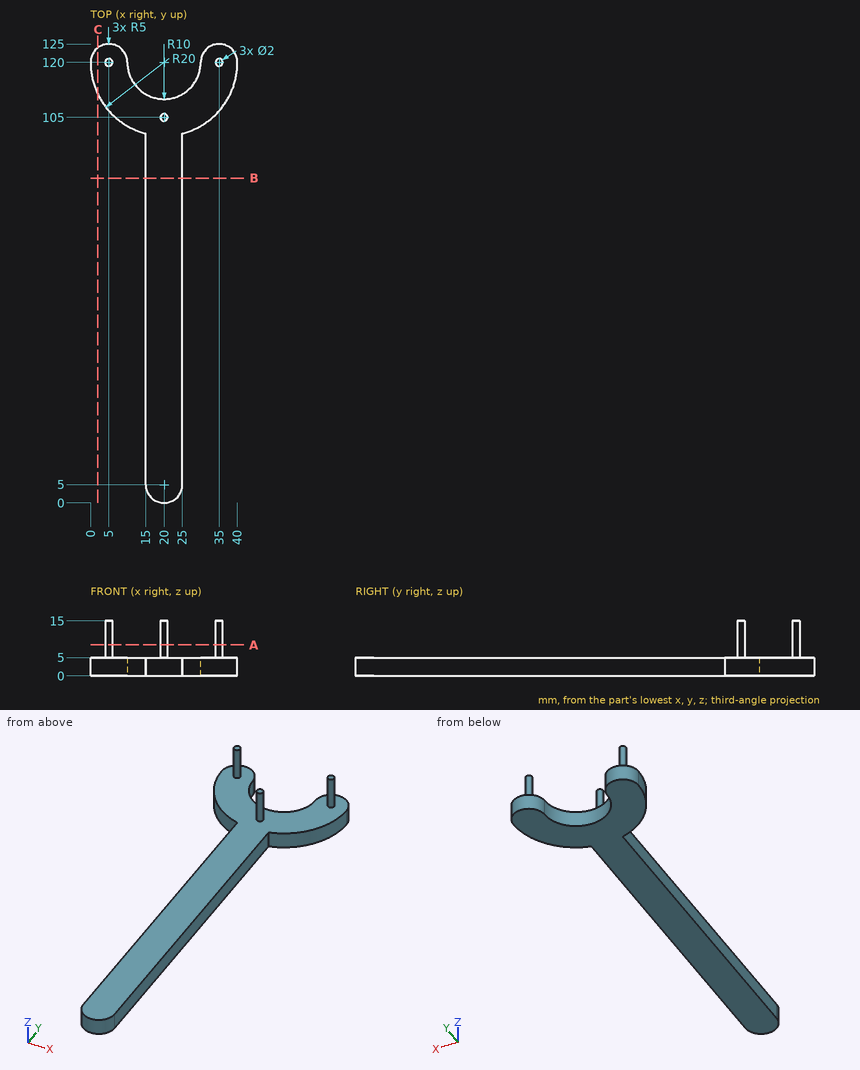
Verification items for this drawing (mm, ordinates from the low corner). Round coordinates to 2 decimals unless told otherwise and drop trailing zeros. Order: outer loops, then holes, each group sorted by start corner. A loop starts at its lowest first (then second) coordinate and runs counter-clockwise, first axis right, second up.
1) Depth check by flat-ended pin: pin 1 (8 mm diameter, centred on x = 28.5, y = 48.5, fed in from +Z); pin 2 (1.5 mm diameter, centred on y = 75, z = 2, fed in from +X); pin 3 (2.5 mm diameter, centred on y = 45.5, z = 2.5, fed in from -X). Enter the tip coordinate at first touch or a pass-through.
Geometry says:
pin 1: stops at z = 5
pin 2: stops at x = 25
pin 3: stops at x = 15
2) Cross-section at C-C, the plane x = 2. Record the cut outline in (y, z), plus the area to 3 significant figures.
Geometry says:
outline: (111.28, 0) - (124, 0) - (124, 5) - (111.28, 5) - close
area: 63.6 mm2
3) Material ranges on line 1 (Z direction, x = 9.5, y = 108); line 2 (X direction, y = 62, z = 1.25); line 3 (Y direction, x = 17, z = 4), recorded low to high.
Geometry says:
line 1: z = 0 to 5
line 2: x = 15 to 25
line 3: y = 1 to 110.46
4) Cross-section at A-A, the plane z = 8.5. Record the cut outline in (x, y).
Geometry says:
outline: circle Ø2 at (5, 120); circle Ø2 at (20, 105); circle Ø2 at (35, 120)
5) Cross-section at B-B, the plane y = 88.5. Record the cut outline in (x, z), plus the area to 3 significant figures.
Geometry says:
outline: (15, 0) - (25, 0) - (25, 5) - (15, 5) - close
area: 50.0 mm2
